Answer from the drawing. Dimensions are ordinates in mm from the lowest x, y and z of the part. A direction names the side the tool comes from. Round coordinates to 2 decimals unless told otherwise and drop trailing zeros. Loops run counter-clockwise (first coordinate to the right, second up) from the corner with the lowest first, then second, coordinate; pieces in that order, holes last. Notation, with made-up numbers: (21.5, 31.5) -> (30.5, 31.5) arc R18 ccw to (30.5, 62.5) -> close; hole circle Ø8 at (83, 60.25). An arc over 180 degrees is marked (long way). Use CSV: the item, a comma, the result in double quotes. Start each with the question number.
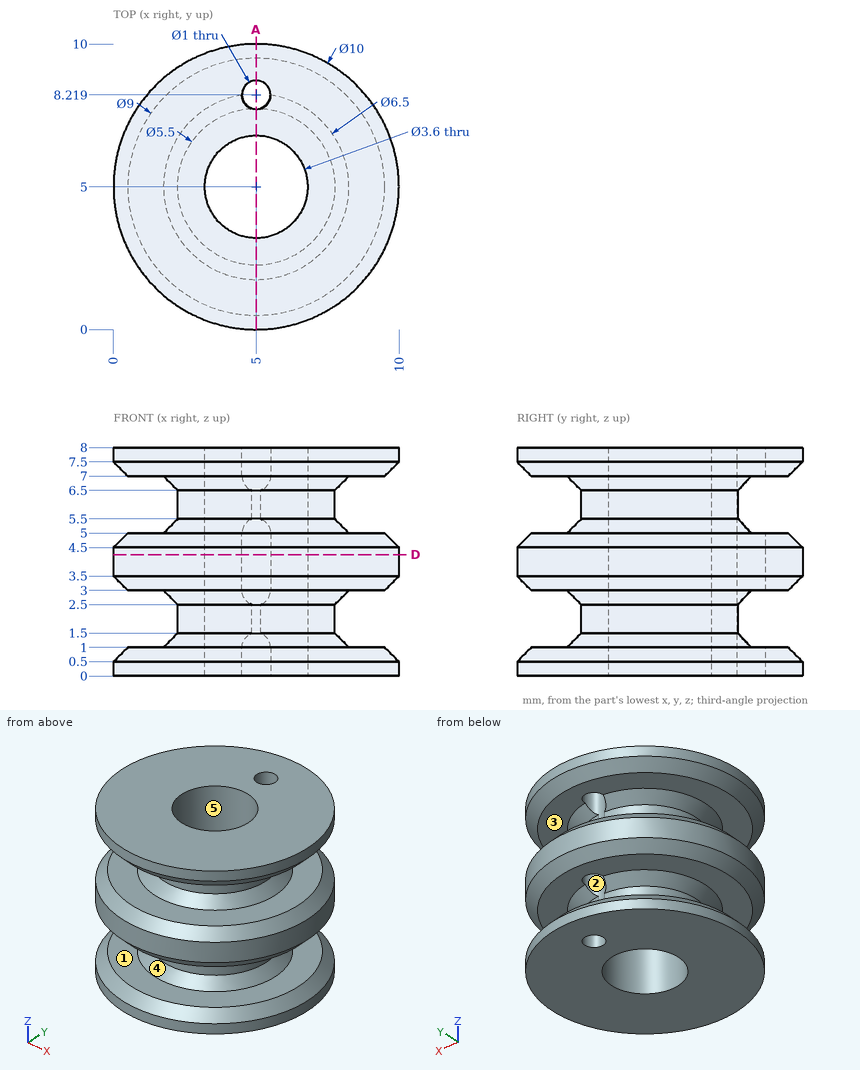
Q1. Section D-D, the plane z = 4.25 is taken. Write down the section's boundary in (x, y).
Q2. Which of the six approach directions +Z, -Z, +X, -X, +Y, -Y give full straight-line access (tool end or side, diameter ignored) to the marked faces 1 and 2?
Q3. Section A-A, the plane x = 5 is taken. Give the number of separate pieces and of enclosed holes in the cut face.
Q4. For a pull along Y with two mould halves and no side action, classify the marked faces 3, 4 and 5 as pulls with the +Y half, pulls with the -Y half, needs draft (parallel to the pull), parting line crosses it, or undercut.
Q5. Each of these flat-tipped pins is pushed along its axis until it touches: pin 1 (2 mm diameter, centred on y = 6.5, z = 1.5, fed in from +X); pin 2 (2 mm diameter, centred on y = 6.5, z = 1.5, fed in from -X); pin 3 (3 mm diameter, centred on y = 8.5, z = 4, fed in from -X). Where does it stop, or does it pass through?
Q6. Straight lines are drawn through the part: line 1 (Z direction, x = 8.5, y = 7.5); line 2 (Z direction, x = 2, y = 1.5); line 3 (Y direction, x = 5, z = 5.25). For each, find the intervals that lie inside material, in ascending order. Write a range as from..to.
Report:
1,outline,"circle Ø10 at (5, 5); hole circle Ø3.6 at (5, 5); hole circle Ø1 at (5, 8.22)"
2,face 1,"none"
2,face 2,"+Z, -Z"
3,separate pieces,"5"
3,enclosed holes,"0"
4,face 3,"needs draft"
4,face 4,"parting line crosses it"
4,face 5,"undercut"
5,pin 1,"stops at x = 9.81"
5,pin 2,"stops at x = 0.19"
5,pin 3,"stops at x = 0.42"
6,line 1,"z = 0..1, 3..5, 7..8"
6,line 2,"z = 0..0.89, 3.11..4.89, 7.11..8"
6,line 3,"y = 2..3.2, 6.8..7.72"
